The model under review builds one solid part; all positions refer to its coordinate system, in mm. A direction names the side the tool comes from. Round coordinates to 2 decimals unless told otherwise and drop trailing zeros. Return JSON: item names as keys, results as strings. Group by question number.
Q1. Draft analysis for pull direction Z (two halves, no side actions). For faces 4 (the face through (-4, -40, 4)), 5 (the face through (-9.76, 42.46, -2.17)), 6 (the face through (-76, 10, -183)), state which applies: pulls with the +Z half, pulls with the -Z half, needs draft (parallel to the pull), parting line crosses it, or undercut.
Q2. To check wall thickness, follow line 1 along X through (y, z) = (17.5, 0); line 2 along X through (y, z) = (1.5, 11); line 3 along Y through (x, z) = (-14.5, -126). State the ranges of each line that lie inside material, in increasing order.
Q3. For faces 1 (the face through (-76, -10, 183)), 2 (the face through (-4.88, 3.09, -1.08)), 3 (the face through (9, 40, 5)), list the 3-axis set-ups (+Z, -Z, +X, -X, +Y, -Y) from which the entire face can be reached by the end or side of a thin tool; tool diameter is ignored.
Q4. Clearance check with flat-ended pins moving along their axes: pin 1 Ø1 at (x, z) = (91.5, -102) entering from +Y; pin 2 Ø10 at (x, y) = (-154, -12.5) entering from -Z; pin 3 Ø10 at (x, z) = (105.5, 41) entering from -Y. State where each tip first meets the part, or that it passes through.
from build123d import *


with BuildPart() as f1:
    # F0 (on Right) → F1 (revolve)
    with BuildSketch(Plane.YZ):
        with BuildLine():
            Line((10, 197), (10, 207.202041))
            ThreePointArc((10, 207.202041), (0, 231), (-10, 207.202041))
            Line((-10, 207.202041), (-10, 197))
            Line((-10, 197), (-1, 194.3))
            Line((-1, 194.3), (-1, 12.658382))
            ThreePointArc((-1, 12.658382), (-20.826062, 14.597093), (-40, 20))
            Line((-40, 20), (-40, 5))
            Line((-40, 5), (40, 5))
            Line((40, 5), (45, 5))
            Line((45, 5), (45, 10))
            Line((45, 10), (40, 10))
            Line((40, 10), (40, 20))
            ThreePointArc((40, 20), (20.826062, 14.597093), (1, 12.658382))
            Line((1, 12.658382), (1, 194.3))
            Line((1, 194.3), (10, 197))
        make_face()
    revolve(axis=Axis((0, 1.765828, 0), (0, 1, 0)))


solid = f1.part
Values:
{
 "1": {"face 4": "needs draft", "face 5": "parting line crosses it", "face 6": "undercut"},
 "2": {"line 1": "x = -14.02 to -5, 5 to 14.02", "line 2": "x = -230.66 to -194.14, -6.27 to 6.27, 194.14 to 230.66", "line 3": "y = -1 to 1"},
 "3": {"face 1": "-Y", "face 2": "+Y, -Y", "face 3": "+Y"},
 "4": {"pin 1": "stops at y = 1", "pin 2": "stops at z = -171.01", "pin 3": "stops at y = -1"}
}
